from build123d import *

# Parameters (mm, degrees)
SKETCH1_W           = 25.4
SKETCH1_H           = 25.4
BOSS_EXTRUDE1_DEPTH = 101.6
SKETCH2_W           = 19.05
SKETCH2_H           = 19.05
CUT_EXTRUDE1_DEPTH  = 102.6
CUT_EXTRUDE2_DEPTH  = 26.4
SKETCH5_R           = 2.4765
CUT_EXTRUDE3_DEPTH  = 26.4
SKETCH7_R           = 4.7625
CUT_EXTRUDE5_DEPTH  = 26.4
SKETCH8_R           = 2.4765
CUT_EXTRUDE6_DEPTH  = 26.4


with BuildPart() as part:
    # Sketch1 → Boss-Extrude1 (new body)
    with BuildSketch(Plane.XY):
        Rectangle(SKETCH1_W, SKETCH1_H)
    extrude(amount=BOSS_EXTRUDE1_DEPTH)

    # Sketch2 → Cut-Extrude1 (cut, through all)
    with BuildSketch(Plane.XY.offset(101.6)):
        Rectangle(SKETCH2_W, SKETCH2_H)
    extrude(amount=-CUT_EXTRUDE1_DEPTH, mode=Mode.SUBTRACT)

    # Sketch4 → Cut-Extrude2 (cut, through all)
    with BuildSketch(Plane(origin=(12.7, 0, 0), x_dir=(0, 0, -1), z_dir=(1, 0, 0))):
        Polygon((-101.6, 12.7), (-76.2, 12.7), (-101.6, -12.7), align=None)
    extrude(amount=-CUT_EXTRUDE2_DEPTH, mode=Mode.SUBTRACT)

    # Sketch5 → Cut-Extrude3 (cut, through all)
    with BuildSketch(Plane.XZ.offset(12.7)):
        with Locations((-6.35, 88.9)):
            Circle(SKETCH5_R)
        with Locations((6.35, 88.9)):
            Circle(SKETCH5_R)
    extrude(amount=-CUT_EXTRUDE3_DEPTH, mode=Mode.SUBTRACT)

    # Sketch7 → Cut-Extrude5 (cut, through all)
    with BuildSketch(Plane(origin=(0, 12.7, 0), x_dir=(1, 0, 0), z_dir=(0, 1, 0))):
        with Locations((0, -12.7)):
            Circle(SKETCH7_R)
    extrude(amount=-CUT_EXTRUDE5_DEPTH, mode=Mode.SUBTRACT)

    # Sketch8 → Cut-Extrude6 (cut, through all)
    with BuildSketch(Plane.XZ.offset(12.7)):
        with Locations((6.35, 31.75)):
            Circle(SKETCH8_R)
        with Locations((-6.35, 31.75)):
            Circle(SKETCH8_R)
    extrude(amount=-CUT_EXTRUDE6_DEPTH, mode=Mode.SUBTRACT)


solid = part.part
Check sheet for the modelled part. Datum: model origin and axes. Units: mm. A direction names the side the tool comes from. Round coordinates to 2 decimals unless told otherwise and drop trailing zeros. Order: outer loops, then holes, each group sorted by start corner. A loop starts at its lowest first (then second) coordinate and runs counter-clockwise, first axis right, second up.
(1) Cross-section at A-A, the plane z = 12.7. Enter the section's corners in (x, y) (1 decimal).
(2) Cross-section at D-D, the plane x = 0. Enter the section's corners in (y, z) (1 decimal), and give its area (3 significant figures).
(3) Scan lines: probe 1 along X at (y, z) = (-1.75, 42) (3 decimals); probe 2 along Z at (x, y) = (-6.35, -10.7). Record each from-to range of solid material in increasing order.
(4) Access from +Z, -Z, +X, -X, +Y, -Y to the whole of each face (thin tool, end or side, straight path). Record for faces 5 (the cylindrical face through (-6.887, 11.09, 29.332)), 6 (the flat face through (-9.525, 0, 50)).
(5) Go/stop test with flat-tipped pins: P1, Ø15, axis at x = 0, z = 12.7, coming from the -Y side; P2, Ø3, axis at x = 6.35, z = 31.75, coming from the -Y side. Record where each tip stops, or that it passes through.
(6) Cross-section at B-B, the plane y = -2.25. Enter the section's corners in (x, z) (3 decimals), and give its area (3 significant figures).
(7) Draft check along X on faces 1 (the cylindrical face through (7.49, -11.13, 86.7)), 2 (the flat face through (12.7, 0, 39)), 3 (the cylindrical face through (5.813, -11.135, 29.332)), 4 (the flat face through (0, 12.7, 38)). Enter one of: pulls with the +X half, pulls with the -X half, needs draft (parallel to the pull), parting line crosses it, or undercut.
(8) Cross-section at C-C, the plane z = 31.75. Enter the section's corners in (x, y) (1 decimal).
Check sheet entries:
1. outline: (-12.7, -12.7) - (-4.8, -12.7) - (-4.8, -9.5) - (-9.5, -9.5) - (-9.5, 9.5) - (-4.8, 9.5) - (-4.8, 12.7) - (-12.7, 12.7) - close; (4.8, -12.7) - (12.7, -12.7) - (12.7, 12.7) - (4.8, 12.7) - (4.8, 9.5) - (9.5, 9.5) - (9.5, -9.5) - (4.8, -9.5) - close
2. outline: (-12.7, 0) - (-9.5, 0) - (-9.5, 7.9) - (-12.7, 7.9) - close; (-12.7, 17.5) - (-9.5, 17.5) - (-9.5, 98.4) - (-12.7, 101.6) - close; (9.5, 0) - (12.7, 0) - (12.7, 7.9) - (9.5, 7.9) - close; (9.5, 17.5) - (12.7, 17.5) - (12.7, 76.2) - (9.5, 79.4) - close
2. area: 504 mm2
3. probe 1: x = -12.7 to -9.525, 9.525 to 12.7
3. probe 2: z = 0 to 29.27, 34.23 to 86.42, 91.38 to 99.6
4. face 5: +Y, -Y
4. face 6: +Z, -Z
5. P1: stops at y = -12.7
5. P2: passes through
6. outline: (-12.7, 0) - (-9.525, 0) - (-9.525, 91.15) - (-12.7, 91.15) - close; (9.525, 0) - (12.7, 0) - (12.7, 91.15) - (9.525, 91.15) - close
6. area: 579 mm2
7. face 1: undercut
7. face 2: pulls with the +X half
7. face 3: undercut
7. face 4: needs draft
8. outline: (-12.7, -12.7) - (-8.8, -12.7) - (-8.8, -9.5) - (-9.5, -9.5) - (-9.5, 9.5) - (-8.8, 9.5) - (-8.8, 12.7) - (-12.7, 12.7) - close; (-3.9, -12.7) - (3.9, -12.7) - (3.9, -9.5) - (-3.9, -9.5) - close; (-3.9, 9.5) - (3.9, 9.5) - (3.9, 12.7) - (-3.9, 12.7) - close; (8.8, -12.7) - (12.7, -12.7) - (12.7, 12.7) - (8.8, 12.7) - (8.8, 9.5) - (9.5, 9.5) - (9.5, -9.5) - (8.8, -9.5) - close
